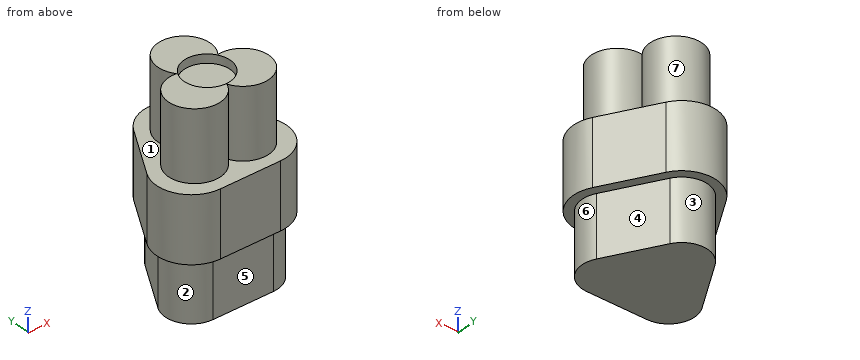
from build123d import *

# Parameters (mm, degrees)
EXTRUDE_1_DEPTH     = 7
EXTRUDE_2_DEPTH     = 7.5
EXTRUDE_3_DEPTH     = 8
SKETCH_4_R          = 2.644424532
CUT_EXTRUDE_1_DEPTH = 1


with BuildPart() as part:
    # ｽｹｯﾁ1 → ﾎﾞｽ - 押し出し1 (new body)
    with BuildSketch(Plane.XY):
        with BuildLine():
            Line((-2.598076211, 5.5), (-6.062177826, -0.5))
            ThreePointArc((-6.062177826, -0.5), (-6.062177826, -3.5), (-3.464101615, -5))
            Line((-3.464101615, -5), (3.464101615, -5))
            ThreePointArc((3.464101615, -5), (6.062177826, -3.5), (6.062177826, -0.5))
            Line((6.062177826, -0.5), (2.598076211, 5.5))
            ThreePointArc((2.598076211, 5.5), (0, 7), (-2.598076211, 5.5))
        make_face()
    extrude(amount=EXTRUDE_1_DEPTH)

    # ｽｹｯﾁ2 → ﾎﾞｽ - 押し出し2 (add)
    with BuildSketch(Plane.XY.offset(7)):
        with BuildLine():
            Line((6.92820323, 0), (3.464101615, 6))
            ThreePointArc((3.464101615, 6), (0, 8), (-3.464101615, 6))
            Line((-3.464101615, 6), (-6.92820323, 0))
            ThreePointArc((-6.92820323, 0), (-6.92820323, -4), (-3.464101615, -6))
            Line((-3.464101615, -6), (3.464101615, -6))
            ThreePointArc((3.464101615, -6), (6.92820323, -4), (6.92820323, 0))
        make_face()
    extrude(amount=EXTRUDE_2_DEPTH)

    # ｽｹｯﾁ3 → ﾎﾞｽ - 押し出し3 (add)
    with BuildSketch(Plane.XY.offset(14.5)):
        with BuildLine():
            ThreePointArc((-2.380628083, 1.374456265), (-5.369357503, -3.1), (0, -2.748912529))
            ThreePointArc((0, -2.748912529), (5.369357503, -3.1), (2.380628083, 1.374456265))
            ThreePointArc((2.380628083, 1.374456265), (0, 6.2), (-2.380628083, 1.374456265))
        make_face()
    extrude(amount=EXTRUDE_3_DEPTH)

    # ｽｹｯﾁ4 → ｶｯﾄ - 押し出し1 (cut)
    with BuildSketch(Plane.XY.offset(22.5)):
        Circle(SKETCH_4_R)
    extrude(amount=-CUT_EXTRUDE_1_DEPTH, mode=Mode.SUBTRACT)


solid = part.part
Source: CAD feature listing. Evaluate the final solid. Frame: model axes, mm. Face numbers are marked on the shaded views. A direction names the side the tool comes from. Give positions to 0.01 mm unless a question says otherwise; leave off trailing zeros. Write each loop counter-clockwise with the first axis right and the second up, starting at its lowest first coordinate (ties: lowest second). Pieces come first, ordered by that corner, then holes. Notation, with made-up numbers: M 20,5.25 L 52,5.25 A14 cw 52,14.25 Z; hole C 16.25,9.5 d4. An arc over 180 degrees is marked long. Answer as a JSON object with one key per item and string values.
Q1. Cut plane C-C, the plane x = -4. Return the cut outline in (y, z).
Geometry check:
{"outline": "M -5.96,7 L -4.95,7 L -4.95,0 L 3.07,0 L 3.07,7 L 5.07,7 L 5.07,14.5 L 1.14,14.5 L 1.14,22.5 L -4.34,22.5 L -4.34,14.5 L -5.96,14.5 Z"}
Q2. Contact query for flat-ended pins moving along their axis: P1, Ø2.5, axis at x = 0, y = -0.5, coming from the +Z side; P2, Ø6, axis at y = 3, z = 6.5, coming from the +X side; P3, Ø5, axis at x = 1, z = 19.5, coming from the -Y side. Output: stop coordinate, or through.
Geometry check:
{"P1": "stops at z = 21.5", "P2": "stops at x = 6.9", "P3": "stops at y = -4.6"}
Q3. Cut plane A-A, the plane z = 6.75. Return the cut outline in (x, y).
Geometry check:
{"outline": "M -6.06,-0.5 A3 ccw -3.46,-5 L 3.46,-5 A3 ccw 6.06,-0.5 L 2.6,5.5 A3 ccw -2.6,5.5 Z"}
Q4. Cut plane B-B, the plane y = 3.5. Return the cut outline in (x, z).
Geometry check:
{"outline": "M -4.91,7 L -3.75,7 L -3.75,0 L 3.75,0 L 3.75,7 L 4.91,7 L 4.91,14.5 L 2.98,14.5 L 2.98,22.5 L -2.98,22.5 L -2.98,14.5 L -4.91,14.5 Z"}
Q5. Cut plane D-D, the plane z = 14. Return the cut outline in (x, y), then the cut area to 3 significant figures.
Geometry check:
{"outline": "M -6.93,0 A4 ccw -3.46,-6 L 3.46,-6 A4 ccw 6.93,0 L 3.46,6 A4 ccw -3.46,6 Z", "area": "154 mm^2"}
Q6. Ray query, line 1 along Z through (x, y) = (3.5, 1.75); line 2 along Y through (x, z) = (-2.5, 16.5); line 3 along X through (y, z) = (4, 2). Return the intervals inside material, ascending.
Geometry check:
{"line 1": "z = 0 to 14.5", "line 2": "y = -4.59 to 1.39, 1.54 to 4.86", "line 3": "x = -3.46 to 3.46"}
Q7. Access query for the marked faces 1, 2, 3 and 4. Directions: +Z, -Z, +X, -X, +Y, -Y. A direction counts if a zero-diameter tool reaches every point of the face in a straight line with its end or side. Return the directions, or none.
Geometry check:
{"face 1": "+Z", "face 2": "-Z, -X", "face 3": "-Z, +Y", "face 4": "-Z, +X, +Y"}
Q8. Mould query, pull axis Y, two halves, no side actions, for the marked faces 5, 6 and 7. Classes: +Y half, -Y half, draft (parallel to the pull), parting line (faces both ways), or undercut.
Geometry check:
{"face 5": "-Y half", "face 6": "parting line", "face 7": "undercut"}
